Autodesk Inventor part; units mm, degrees
ref_plane "YZ Plane" through (0, 0, 0) normal (1, 0, 0) x (0, 1, 0)
ref_plane "XZ Plane" through (0, 0, 0) normal (0, 1, 0) x (-1, 0, 0)
ref_plane "XY Plane" through (0, 0, 0) normal (0, 0, 1) x (1, 0, 0)
sketch "Sketch2" plane through (0, 0, 0) normal (0, 1, 0) x (-1, 0, 0)
  line L0 (30, 30) -> (-30, 30)
  line L1 (-30, 30) -> (-30, -30)
  line L2 (-30, -30) -> (30, -30)
  line L3 (30, -30) -> (30, 30)
  line L4 (30, 30) -> (-30, -30) construction
  line L5 (-30, 30) -> (30, -30) construction
  line L6 (-28, -28) -> (-28, 28)
  line L7 (-28, 28) -> (28, 28)
  line L8 (28, 28) -> (28, -28)
  line L9 (28, -28) -> (-28, -28)
  point P0 (0, 0)
  point P1 (0, -190)
  point P2 (0, 0)
  dimension "d6" = 60
  dimension "d49" = 2
extrude "Extrusion2" add sketch "Sketch2" along normal blind 2100
sketch "Sketch6" plane through (30, 0, -30) normal (0, 0, -1) x (-1, 0, 0)
  line L0 (0, 0) -> (60, 0)
  line L1 (60, 0) -> (60, 2100) construction
  line L2 (0, 2100) -> (60, 2100)
  line L3 (0, 0) -> (0, 2100) construction
  circle A0 centre (44, 60) radius 10.5
  circle A1 centre (16, 360) radius 10.5
  point P0 (30, 0)
  dimension "d44" = 21
  dimension "d45" = 16
  dimension "d46" = 16
  dimension "d47" = 300
  dimension "d48" = 60
extrude "Extrusion6" cut sketch "Sketch6" against normal up to surface (2 mm away)
pattern_linear "Rectangular Pattern2" count 8 spacing 240 along (0, 1, 0) of "Extrusion6"
equation "\"d46\" = d45"
properties part number "DMF 082 коллектор болванка"
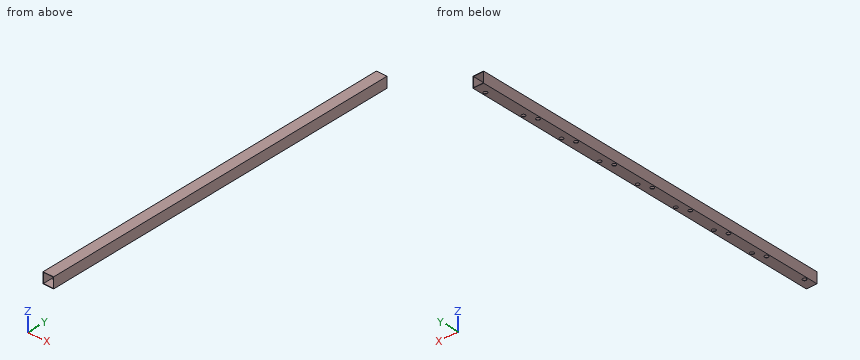
Design review of the part built by this model. Coordinates are the model's own, in mm. Coordinates: 2 decimals unless noted, no trailing zeros. Loops run counter-clockwise (first coordinate to the right, second up) from the corner with the lowest first, then second, coordinate; pieces in that order, holes last. Notation, with made-up numbers: M 13.25,6.5 L 56.25,6.5 A32 cw 56.25,37.5 Z; hole C -23,23 d9. An arc over 180 degrees is marked long. Answer as CSV lines item,"result".
Item 1: Add section A-A on z = -8. State the section outline as (x, y) points.
Answer list:
outline,"M -30,0 L -28,0 L -28,2100 L -30,2100 Z; M 28,0 L 30,0 L 30,2100 L 28,2100 Z"
Item 2: Add section B-B on y = 1408. State the section outline as (x, z) points, plus the area to 3 significant figures.
Answer list:
outline,"M -30,-30 L 30,-30 L 30,30 L -30,30 Z; hole M -28,-28 L 28,-28 L 28,28 L -28,28 Z"
area,"464 mm²"
Item 3: For probe 1 along Z at (x, y) = (-14.5, 1886.5); probe 2 along X at (y, z) = (1560, -29.2), list the stretches that pass through material, from the lowest coordinate up.
Answer list:
probe 1,"-30 to -28, 28 to 30"
probe 2,"-30 to 3.5, 24.5 to 30"
Item 4: For P1, Ø19, axis at x = -14, y = 1020, coming from the -Z side, flat-tipped, find the tip position at first contact; note if it passes through.
Answer list:
P1,"z = 28"
